Check sheet for the modelled part. Datum: model origin and axes. Units: mm. A direction names the side the tool comes from. Round coordinates to 2 decimals unless told otherwise and drop trailing zeros. Order: outer loops, then holes, each group sorted by start corner. A loop starts at its lowest first (then second) coordinate and runs counter-clockwise, first axis right, second up. Notation, with made-up numbers: (9.5, 1.25) -> (43.5, 1.25) arc R16 ccw to (43.5, 21.25) -> close; hole circle Ø1 at (34, 83.25). An arc over 180 degrees is marked (long way). Use CSV: the item, a comma, the result in double quotes.
```python
from build123d import *

# Parameters (mm, degrees)
SKETCH_2_R          = 1.5
EXTRUDE_1_DEPTH     = 6
CUT_EXTRUDE_1_DEPTH = 2
CHAMFER_1_SIZE      = 0.2
FILLET_1_R          = 0.2


with BuildPart() as part:
    # 草图1 → 旋转1 (revolve)
    with BuildSketch(Plane.XY):
        Polygon((0, 0), (0, -2), (1.5, -2), (3, 0), align=None)
    revolve(axis=Axis((0, 0, 0), (0, -1, 0)))

    # 草图2 → 凸台-拉伸1 (add)
    with BuildSketch(Plane.XZ.offset(2)):
        Circle(SKETCH_2_R)
    extrude(amount=EXTRUDE_1_DEPTH)

    # 草图3 → 切除-拉伸1 (cut)
    with BuildSketch(Plane(origin=(0, 0, 0), x_dir=(1, 0, 0), z_dir=(0, 1, 0))):
        Polygon((-1.327905619, 0), (-0.66395281, -1.15), (0.66395281, -1.15), (1.327905619, 0), (0.66395281, 1.15), (-0.66395281, 1.15), align=None)
    extrude(amount=-CUT_EXTRUDE_1_DEPTH, mode=Mode.SUBTRACT)

    # 倒角1
    chamfer_1_edges = [part.edges().sort_by_distance(p)[0] for p in [
        (-1.5, -8, 0),
    ]]
    chamfer(chamfer_1_edges, length=CHAMFER_1_SIZE)

    # 圆角1
    fillet_1_edges = [part.edges().sort_by_distance(p)[0] for p in [
        (-3, 0, 0),
    ]]
    fillet(fillet_1_edges, radius=FILLET_1_R)


solid = part.part
```
Q1. Sectioned sample at A-A, the plane x = 0. Enter the section's corners in (y, z).
Result sheet:
outline,"(-8, -1.3) -> (-7.8, -1.5) -> (-2, -1.5) -> (-0.32, -2.76) arc R0.2 ccw to (0, -2.6) -> (0, -1.15) -> (-2, -1.15) -> (-2, 1.15) -> (0, 1.15) -> (0, 2.6) arc R0.2 ccw to (-0.32, 2.76) -> (-2, 1.5) -> (-7.8, 1.5) -> (-8, 1.3) -> close"
Q2. Sectioned sample at B-B, the plane y = -0.5. Enter the section's corners in (x, z) (3 decimals).
Result sheet:
outline,"circle Ø5.25 at (0, 0); hole (-1.328, 0) -> (-0.664, -1.15) -> (0.664, -1.15) -> (1.328, 0) -> (0.664, 1.15) -> (-0.664, 1.15) -> close"
Q3. Access from +Z, -Z, +X, -X, +Y, -Y to the whole of each face (thin tool, end or side, straight path). Record for faces 1 (the face through (1, 0, -1)), 2 (the face through (0.991, -0.986, 0.583)).
Result sheet:
face 1,"+Z, -Z, +X, -X, +Y"
face 2,"+Y"
Q4. Scan lines: L1, parallel to Y at x = 0.6, z = -0.7; L2, parallel to Z at x = 0.75, y = -0.5; L3, parallel to Y at x = -1.95, z = -0.55. Record each from-to range of solid material in increasing order.
Result sheet:
L1,"y = -8 to -2"
L2,"z = -2.52 to -1, 1 to 2.52"
L3,"y = -1.3 to 0"
Q5. Mould release check, pull along X, two halves, no side actions. Record for faces 3 (the face through (-0.991, -0.986, -0.583)), 4 (the face through (-1.5, -4.86, 0.07)), 5 (the face through (0, -8, 0)), 6 (the face through (0, -2, 0)): pulls with the +X half, pulls with the -X half, needs draft (parallel to the pull), parting line crosses it, or undercut.
Result sheet:
face 3,"undercut"
face 4,"parting line crosses it"
face 5,"needs draft"
face 6,"undercut"
Q6. Sectioned sample at C-C, the plane y = -4. Enter the section's corners in (x, z), then the cut area to 3 significant figures.
Result sheet:
outline,"circle Ø3 at (0, 0)"
area,"7.07 mm^2"
Q7. Go/stop test with flat-tipped pins: pin 1 (1.5 mm diameter, centred on x = 0.5, y = -1, fed in from +Z); pin 2 (3 mm diameter, centred on y = -4, z = 1.5, fed in from +X); pin 3 (1 mm diameter, centred on y = -3.5, z = 1, fed in from -X). Record where each tip stops, or that it passes through.
Result sheet:
pin 1,"stops at z = 2.77"
pin 2,"stops at x = 1.5"
pin 3,"stops at x = -1.41"
